The listing builds one solid part. Answer for the finished solid, in the listing's coordinates (mm). Face numbers are marked on the shaded views. A direction names the side the tool comes from. Give positions to 0.01 mm unless a question says otherwise; leave off trailing zeros. Loops run counter-clockwise (first coordinate to the right, second up) from the corner with the lowest first, then second, coordinate; pieces in that order, holes last. Notation, with made-up numbers: (72.5, -21) - (87.5, -21) arc R18 ccw to (87.5, 12) - close; hole circle Ø3 at (-9, 55.25). An arc over 180 degrees is marked (long way). Answer as CSV lines item,"result". Start each with the question number.
1) A cutting plane is placed at A-A (y = 0). Determine the outline of the cut face in (x, z), and give its area (3 significant figures).
2) Flat-ended cylindrical pins translate along their axes: pin 1 (2 mm diameter, centred on y = 1.5, z = 15, fed in from -X); pin 2 (2 mm diameter, centred on x = 0.5, y = 0.5, fed in from +Z). Find the tip coordinate at first contact, or state that the pin passes through.
3) A cutting plane is placed at C-C (z = 35). Determine the outline of the cut face in (x, y).
4) For the marked faces 1 and 2, determine the directions among +Z, -Z, +X, -X, +Y, -Y from which every point of the face is accessible in a straight line to the end or side of a thin tool.
5) Find the intervals of material crossed by line 1 along Y through (x, z) = (0, 23.5); line 2 along Z through (x, y) = (-1.3, -0.4); line 3 along Y through (x, z) = (-2, 27), in increasing order.
```python
from build123d import *

# Parameters (mm, degrees)
SKETCH_1_R      = 2.5
SKETCH_1_R_2    = 1.4
EXTRUDE_1_DEPTH = 40
SKETCH_2_R      = 1.5
EXTRUDE_2_DEPTH = 6


with BuildPart() as part:
    # 草图1 → 凸台-拉伸1 (new body)
    with BuildSketch(Plane.XY):
        Circle(SKETCH_1_R)
        Circle(SKETCH_1_R_2, mode=Mode.SUBTRACT)
    extrude(amount=EXTRUDE_1_DEPTH)

    # 草图2 → 凸台-拉伸2 (add)
    with BuildSketch(Plane(origin=(0, 0, 0), x_dir=(-1, 0, 0), z_dir=(0, 0, -1))):
        with Locations(Location((0, 0, 0), (0, 0, 180))):
            Circle(SKETCH_2_R)
    extrude(amount=EXTRUDE_2_DEPTH)


solid = part.part
```
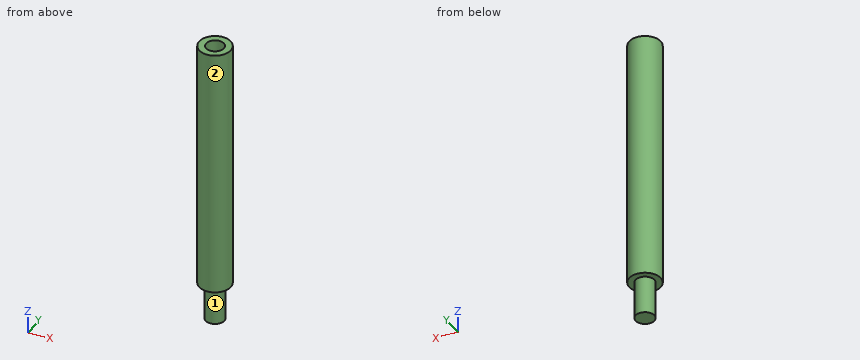
Ans:
1,outline,"(-2.5, 0) - (-1.5, 0) - (-1.5, -6) - (1.5, -6) - (1.5, 0) - (2.5, 0) - (2.5, 40) - (1.4, 40) - (1.4, 0) - (-1.4, 0) - (-1.4, 40) - (-2.5, 40) - close"
1,area,"106 mm2"
2,pin 1,"x = -2.45"
2,pin 2,"z = 40"
3,outline,"circle Ø5 at (0, 0); hole circle Ø2.8 at (0, 0)"
4,face 1,"-Z"
4,face 2,"+Z, -Z"
5,line 1,"-2.5 to -1.4, 1.4 to 2.5"
5,line 2,"-6 to 0"
5,line 3,"-1.5 to 1.5"
